Geometry check sheet. Reference: the model listing, model coordinates, mm. Face numbers are marked on the shaded views. A direction names the side the tool comes from. Round coordinates to 2 decimals unless told otherwise and drop trailing zeros. Write each loop counter-clockwise with the first axis right and the second up, starting at its lowest first coordinate (ties: lowest second). Pieces come first, ordered by that corner, then holes. Notation, with made-up numbers: (50.25, 11.5) - (84.25, 11.5) arc R23 ccw to (84.25, 45.5) - close; hole circle Ø9 at (20.25, 40). An arc over 180 degrees is marked (long way). Return JSON: item names as keys, results as strings. Group by question number.
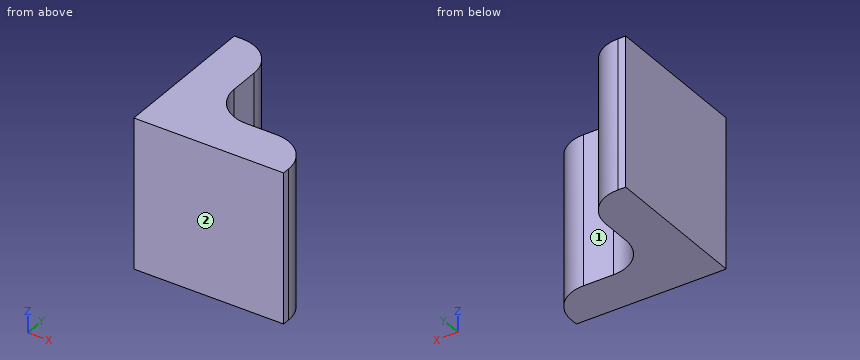
from build123d import *

# Parameters (mm, degrees)
F1_DEPTH = 25.4


with BuildPart() as f1:
    # F0 (on Top) → F1 (new body)
    with BuildSketch(Plane.XY):
        with BuildLine():
            Line((1.27, 25.4), (0, 25.4))
            Line((0, 25.4), (0, 0))
            Line((0, 0), (25.4, 0))
            Line((25.4, 0), (25.4, 1.27))
            ThreePointArc((25.4, 1.27), (23.540128, 5.760128), (19.05, 7.62))
            Line((19.05, 7.62), (13.97, 7.62))
            ThreePointArc((13.97, 7.62), (9.479872, 9.479872), (7.62, 13.97))
            Line((7.62, 13.97), (7.62, 19.05))
            ThreePointArc((7.62, 19.05), (5.760128, 23.540128), (1.27, 25.4))
        make_face()
    extrude(amount=F1_DEPTH)


solid = f1.part
1. Section check B-B (x = 18). Enter the section's corners in (y, z), and give its area (3 significant figures).
2. Material ranges on line 1 along X through (y, z) = (19.25, 15.25); line 2 along Y through (x, z) = (6, 3.75), recorded low to high.
3. Section check A-A (z = 9.5). Enter the section's corners in (x, y).
4. Depth check by flat-ended pin: pin 1 Ø3 at (x, z) = (10.5, 14) entering from +Y; pin 2 Ø4 at (x, z) = (13.5, 2.5) entering from +Y; pin 3 Ø4 at (x, y) = (10, 7.5) entering from -Z; pin 4 Ø4 at (y, z) = (15.5, 12.5) entering from +X. Enter the tip coordinate at first touch or a pass-through.
5. Section check C-C (y = 21). Enter the section's corners in (x, z), and give its area (3 significant figures).
6. Tool access check on the marked faces 1 and 2. Record the directions out of +Z, -Z, +X, -X, +Y, -Y that give a thin tool (end or side, any length) a straight path to the whole face; none if there is none.
Result sheet:
{
 "1": {"outline": "(0, 0) - (7.62, 0) - (7.62, 25.4) - (0, 25.4) - close", "area": "194 mm²"},
 "2": {"line 1": "x = 0 to 7.62", "line 2": "y = 0 to 23.29"},
 "3": {"outline": "(0, 0) - (25.4, 0) - (25.4, 1.27) arc R6.35 ccw to (19.05, 7.62) - (13.97, 7.62) arc R6.35 cw to (7.62, 13.97) - (7.62, 19.05) arc R6.35 ccw to (1.27, 25.4) - (0, 25.4) - close"},
 "4": {"pin 1": "stops at y = 10.02", "pin 2": "stops at y = 8.12", "pin 3": "stops at z = 0", "pin 4": "stops at x = 7.64"},
 "5": {"outline": "(0, 0) - (7.31, 0) - (7.31, 25.4) - (0, 25.4) - close", "area": "186 mm²"},
 "6": {"face 1": "+Z, -Z, +X, +Y", "face 2": "+Z, -Z, +X, -X, -Y"}
}
